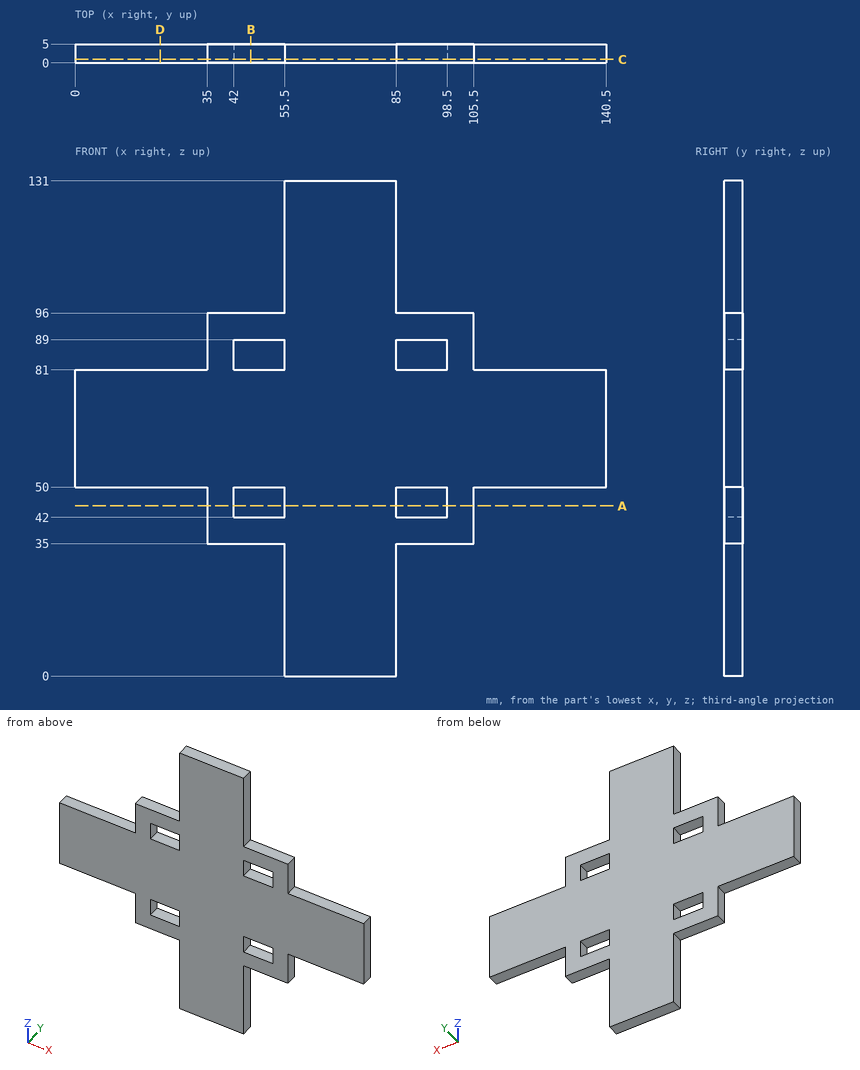
Check sheet for the drawn part. Datum: minimum x, y, z corner. Units: mm. Coordinates: 2 decimals unless noted, no trailing zeros. Loops run counter-clockwise (first coordinate to the right, second up) from the corner with the lowest first, then second, coordinate; pieces in that order, holes last. Notation, with made-up numbers: (6.5, 19) -> (41.5, 19) arc R14 ccw to (41.5, 31) -> close; hole circle Ø2 at (52, -33). An arc over 180 degrees is marked (long way). Answer as a JSON object with one key per item and string values. Group by question number.
Item 1: Sectioned sample at C-C on y = 0.95. State how many separate pieces and enclosed holes the cut face has, plus the area to 3 significant figures.
Item 2: Scan lines: probe 1 along X at (y, z) = (2, 47.5); probe 2 along Z at (x, y) = (46.5, 2.25); probe 3 along Z at (x, y) = (100, 4.3). Record each from-to range of solid material in increasing order.
Item 3: Sectioned sample at D-D on x = 22.5. Record the boundary of the cut face in (y, z), plus the area to 3 significant figures.
Item 4: Sectioned sample at B-B on x = 46.5. Record the boundary of the cut face in (y, z).
Item 5: Depth check by flat-ended pin: pin 1 (2.5 mm diameter, centred on x = 51.5, y = 2.5, fed in from +Z); pin 2 (1.5 mm diameter, centred on x = 14.5, y = 3, fed in from -Z); pin 3 (1.5 mm diameter, centred on y = 2, z = 14, fed in from +X). Enter the tip coordinate at first touch or a pass-through.
Item 6: Sectioned sample at A-A on z = 45. Record the boundary of the cut face in (x, y), plus the area to 4 significant figures.
Evaluation:
{
 "1": {"separate pieces": "1", "enclosed holes": "4", "area": "8,100 mm²"},
 "2": {"probe 1": "x = 35 to 42, 55.5 to 85, 98.5 to 105.5", "probe 2": "z = 35 to 42, 50 to 81, 89 to 96", "probe 3": "z = 35 to 96"},
 "3": {"outline": "(0, 50) -> (5, 50) -> (5, 81) -> (0, 81) -> close", "area": "155 mm²"},
 "4": {"outline": "(0, 35) -> (5, 35) -> (5, 42) -> (0, 42) -> close; (0, 50) -> (5, 50) -> (5, 81) -> (0, 81) -> close; (0, 89) -> (5, 89) -> (5, 96) -> (0, 96) -> close"},
 "5": {"pin 1": "stops at z = 96", "pin 2": "stops at z = 50", "pin 3": "stops at x = 85"},
 "6": {"outline": "(35, 0) -> (42, 0) -> (42, 5) -> (35, 5) -> close; (55.5, 0) -> (85, 0) -> (85, 5) -> (55.5, 5) -> close; (98.5, 0) -> (105.5, 0) -> (105.5, 5) -> (98.5, 5) -> close", "area": "217.5 mm²"}
}
